Source: three-view drawing plus pictorial views. Frame: mm from the lowest corner of the part. Round coordinates to 2 decimals unless told otherwise and drop trailing zeros. Write each loop counter-clockwise with the first axis right and the second up, starting at its lowest first coordinate (ties: lowest second). Pieces come first, ordered by that corner, then holes.
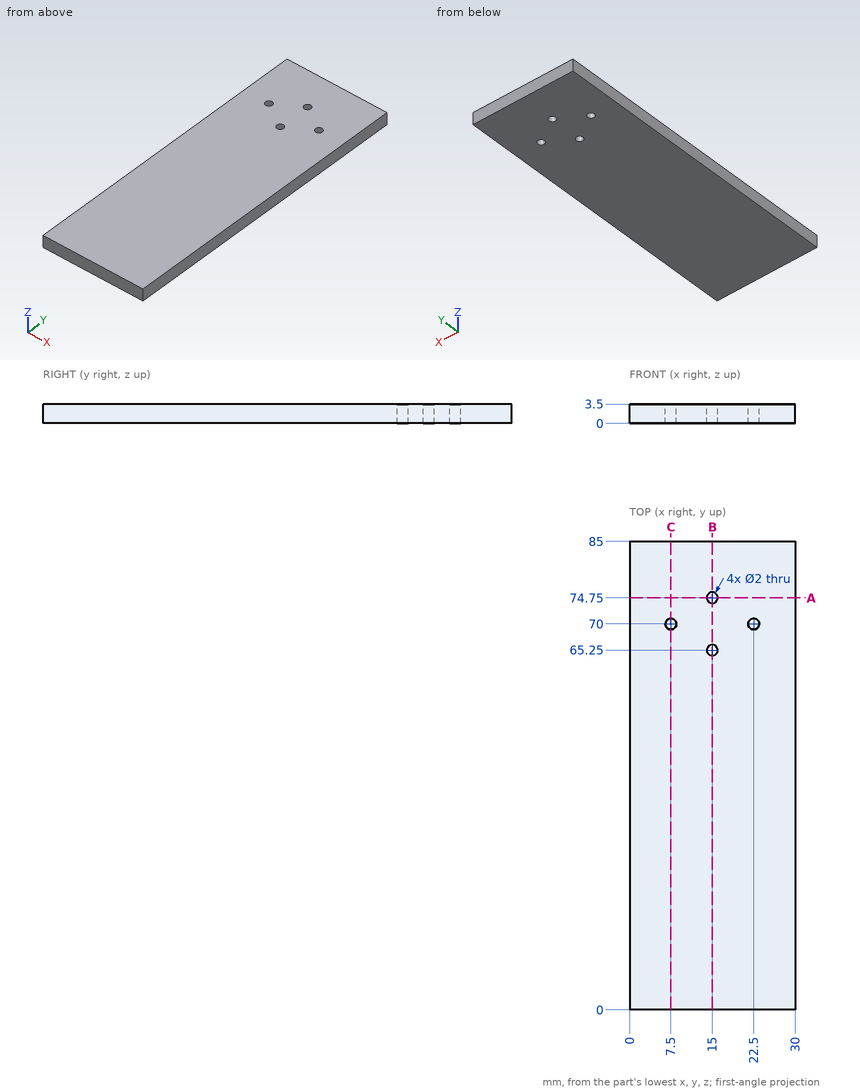
1) Line query: probe 1 along X at (y, z) = (70, 0.9); probe 2 along X at (y, z) = (65.25, 2.5); probe 3 along Y at (x, z) = (15.5, 1.75). Output: solid intervals per line, ascending.
2) Section A-A on y = 74.75. Output: boundary loops of the cut face in (x, z), plus the area to 3 significant figures.
3) Section C-C on x = 7.5. Output: boundary loops of the cut face in (y, z), plus the area to 4 significant figures.
4) Section B-B on x = 15. Output: boundary loops of the cut face in (y, z).
Filled in:
1. probe 1: x = 0 to 6.5, 8.5 to 21.5, 23.5 to 30
1. probe 2: x = 0 to 14, 16 to 30
1. probe 3: y = 0 to 64.38, 66.12 to 73.88, 75.62 to 85
2. outline: (0, 0) - (14, 0) - (14, 3.5) - (0, 3.5) - close; (16, 0) - (30, 0) - (30, 3.5) - (16, 3.5) - close
2. area: 98.0 mm2
3. outline: (0, 0) - (69, 0) - (69, 3.5) - (0, 3.5) - close; (71, 0) - (85, 0) - (85, 3.5) - (71, 3.5) - close
3. area: 290.5 mm2
4. outline: (0, 0) - (64.25, 0) - (64.25, 3.5) - (0, 3.5) - close; (66.25, 0) - (73.75, 0) - (73.75, 3.5) - (66.25, 3.5) - close; (75.75, 0) - (85, 0) - (85, 3.5) - (75.75, 3.5) - close
